Autodesk Inventor part; units mm, degrees
ref_plane "YZ Plane" through (0, 0, 0) normal (1, 0, 0) x (0, 1, 0)
ref_plane "XZ Plane" through (0, 0, 0) normal (0, 1, 0) x (-1, 0, 0)
ref_plane "XY Plane" through (0, 0, 0) normal (0, 0, 1) x (1, 0, 0)
sketch "Skizze1" plane through (0, 0, 0) normal (0, 0, 1) x (1, 0, 0)
  line L0 (0, 0) -> (0, 17.5)
  line L1 (0, 17.5) -> (5, 17.5)
  line L2 (5, 17.5) -> (5, 20)
  line L3 (5, 20) -> (55, 20)
  line L4 (55, 20) -> (55, 0)
  line L5 (55, 0) -> (0, 0)
  line L6 (0, 11) -> (7, 11)
  line L7 (7, 11) -> (7, 8)
  line L8 (7, 8) -> (48, 8)
  line L9 (48, 8) -> (48, 11)
  line L10 (48, 11) -> (55, 11)
  line L11 (5, 20) -> (12, 20)
  line L12 (12, 20) -> (12, 30)
  line L13 (12, 30) -> (5, 30)
  line L14 (5, 30) -> (5, 20)
  dimension "d1" = 17.5
  dimension "d2" = 5
  dimension "d4" = 50
  dimension "d5" = 8
  dimension "d6" = 11
  dimension "d7" = 7
  dimension "d8" = 7
  dimension "d31" = 20
  dimension "d32" = 7
  dimension "d33" = 30
revolve "Umdrehung1" add sketch "Skizze1" angle 360 about axis through (55, 0, 0) along (-1, 0, 0) contours L0 L1 L2 L3 L4 L10 L9 L8 L7 L6 | L14 L13 L12 L3
sketch "Skizze4" plane through (55, 0, 0) normal (1, 0, 0) x (0, 0, -1)
  circle A0 centre (0, 0) radius 15.5
  circle A1 centre (0, 0) radius 11
  circle A2 centre (0, 0) radius 20
  line L0 (10.9602, 10.9602) -> (10.9602, -10.9602)
  line L1 (10.9602, -10.9602) -> (-10.9602, -10.9602)
  line L2 (-10.9602, -10.9602) -> (-10.9602, 10.9602)
  line L3 (-10.9602, 10.9602) -> (10.9602, 10.9602)
  dimension "d20" = 4.5
  dimension "d21" = 4.5
hole "Bohrung2" at (55, 10.9602, -10.9602) at (55, -10.9602, -10.9602) at (55, -10.9602, 10.9602) at (55, 10.9602, 10.9602) direction (-1, 0, 0) diameter 3.242 depth 10 tip angle 118
sketch "Skizze6" plane through (5, 0, 0) normal (-1, 0, 0) x (0, 0, 1)
  circle A0 centre (0, 0) radius 24
  line L0 (-16.9706, 16.9706) -> (16.9706, 16.9706)
  line L1 (16.9706, 16.9706) -> (16.9706, -16.9706)
  line L2 (16.9706, -16.9706) -> (-16.9706, -16.9706)
  line L3 (-16.9706, -16.9706) -> (-16.9706, 16.9706)
  dimension "d34" = 48
hole "Bohrung3" at (5, 16.9706, -16.9706) at (5, -16.9706, -16.9706) at (5, -16.9706, 16.9706) at (5, 16.9706, 16.9706) direction (1, 0, 0) diameter 4.917 depth 17.1 tip angle 118
equation "\"d20\" = d21"
properties part number "Lagerhalter"
Part model, mm, in its own coordinate system. A direction names the side the tool comes from. Coordinates: 2 decimals unless noted, no trailing zeros. Loops run counter-clockwise (first coordinate to the right, second up) from the corner with the lowest first, then second, coordinate; pieces in that order, holes last. Notation, with made-up numbers: (-6, 26.5) - (1, 26.5) arc R23 cw to (1, 53.5) - close; hole circle Ø7 at (7, 79.5). An arc over 180 degrees is marked (long way). Write item = value, one per line. Start each with the question number.
Item 1: Flat gauge pins, fed straight in: pin 1 Ø2 at (x, y) = (45.5, 1) entering from +Z; pin 2 Ø10 at (x, y) = (42, -9) entering from -Z; pin 3 Ø9.5 at (y, z) = (0, 0) entering from -X (1 decimal); pin 4 Ø17.5 at (y, z) = (0, 0) entering from +X. Where does each tip first touch, or does it go through?
Item 2: Cut at C-C, the plane x = 20. Give the cut face in (y, z), and give its area (3 significant figures).
Item 3: Wall check: L1, parallel to Y at x = 50, z = 0; L2, parallel to Z at x = 32, y = 0; L3, parallel to X at y = -27, z = -10. Give the ranges that are in metal, low to high. Write a range as from..to.
Item 4: Cut at D-D, the plane z = -23. Give the cut face in (x, y).
Item 5: Cut at A-A, the plane z = 0. Give the cut face in (x, y), and give its area (3 significant figures).
Item 6: Mould opens along Z. For faces 1 (the flat face through (48, -2, 8)), 2 (the cylindrical face through (2.535, -13.887, -10.648)), 3 (the flat face through (55, 9, 9)) say: released by +Z, released by -Z, zero draft, split by the parting line, or undercut.
Item 7: 3-axis set-ups, long thin cutter, end or side, ignore diameter. For faces 4 (the cylindrical face through (49.93, -9.378, 11.312)), 5 (the cylindrical face through (8.549, 16.232, 19.316)), 6 (the flat face through (7, -2, 8)): which of +Z, -Z, +X, -X, +Y, -Y reach the whole face in a straight line?
The answers:
q1.pin_1 = 20
q1.pin_2 = -19.6
q1.pin_3 = through
q1.pin_4 = 48
q2.outline = circle Ø40 at (0, 0); hole circle Ø16 at (0, 0)
q2.area = 1,060 mm2
q3.L1 = -20..-11, 11..20
q3.L2 = -20..-8, 8..20
q3.L3 = 5..12
q4.outline = (5, -19.26) - (12, -19.26) - (12, 19.26) - (5, 19.26) - close
q5.outline = (0, -17.5) - (5, -17.5) - (5, -30) - (12, -30) - (12, -20) - (55, -20) - (55, -11) - (48, -11) - (48, -8) - (7, -8) - (7, -11) - (0, -11) - close; (0, 11) - (7, 11) - (7, 8) - (48, 8) - (48, 11) - (55, 11) - (55, 20) - (12, 20) - (12, 30) - (5, 30) - (5, 17.5) - (0, 17.5) - close
q5.area = 1,350 mm2
q6.face_1 = undercut
q6.face_2 = split by the parting line
q6.face_3 = zero draft
q7.face_4 = +X
q7.face_5 = +X, -X
q7.face_6 = -X
